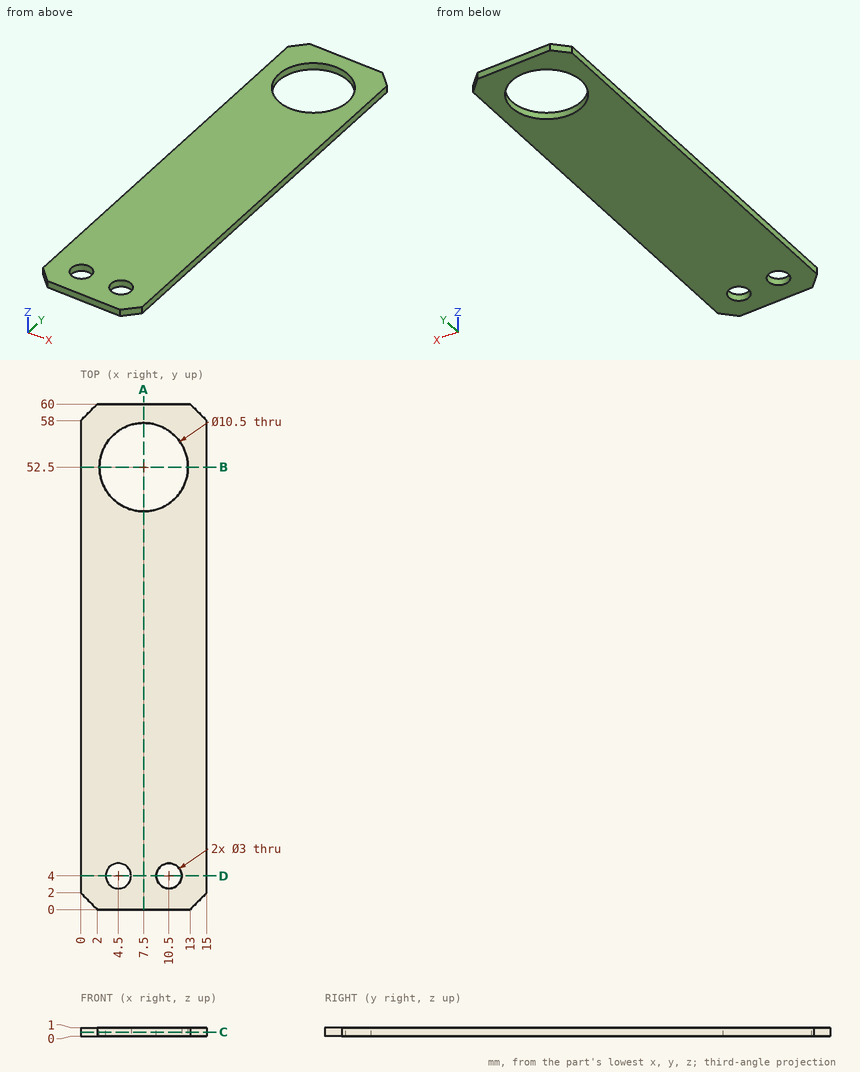
Can you work these out from the drawing? Everything is in mm from the part's minimum corner. Give positions to 0.01 mm unless a question says otherwise; leave off trailing zeros. Order: outer loops, then holes, each group sorted by start corner. A loop starts at its lowest first (then second) coordinate and runs counter-clockwise, first axis right, second up. Notation, with made-up numbers: (45.5, 88.5) -> (79.5, 88.5) arc R16 ccw to (79.5, 107.5) -> close; hole circle Ø2 at (52, 42.25). An arc over 180 degrees is marked (long way). Return JSON: item names as keys, results as strings.
1. Imagine slicing it at D-D on y = 4. List the corners of the cut face in (x, z) for me, then the cut area to 3 significant figures.
Answer list:
{"outline": "(0, 0) -> (3, 0) -> (3, 1) -> (0, 1) -> close; (6, 0) -> (9, 0) -> (9, 1) -> (6, 1) -> close; (12, 0) -> (15, 0) -> (15, 1) -> (12, 1) -> close", "area": "9.00 mm2"}
2. Imagine slicing it at B-B on y = 52.5. List the corners of the cut face in (x, z) for me, then the cut area to 3 significant figures.
Answer list:
{"outline": "(0, 0) -> (2.25, 0) -> (2.25, 1) -> (0, 1) -> close; (12.75, 0) -> (15, 0) -> (15, 1) -> (12.75, 1) -> close", "area": "4.50 mm2"}
3. Imagine slicing it at A-A on x = 7.5. List the corners of the cut face in (y, z) for me.
Answer list:
{"outline": "(0, 0) -> (47.25, 0) -> (47.25, 1) -> (0, 1) -> close; (57.75, 0) -> (60, 0) -> (60, 1) -> (57.75, 1) -> close"}
4. I need wall thicknesses on line 1 (Y direction, x = 10.5, z = 0.3); line 2 (Y direction, x = 4.75, z = 0.75); line 3 (X direction, y = 52.5, z = 0.4). Which ranges of each line are inside material? Lowest first, please. Write a range as from..to.
Answer list:
{"line 1": "y = 0..2.5, 5.5..48.19, 56.81..60", "line 2": "y = 0..2.52, 5.48..48.03, 56.97..60", "line 3": "x = 0..2.25, 12.75..15"}
5. Imagine slicing it at C-C on z = 0.45. List the corners of the cut face in (x, y) for me, then the cut area to 3 significant figures.
Answer list:
{"outline": "(0, 2) -> (2, 0) -> (13, 0) -> (15, 2) -> (15, 58) -> (13, 60) -> (2, 60) -> (0, 58) -> close; hole circle Ø10.5 at (7.5, 52.5); hole circle Ø3 at (4.5, 4); hole circle Ø3 at (10.5, 4)", "area": "791 mm2"}
